Build history of the part. All positions in model axes, mm. A direction names the side the tool comes from. Coordinates: 2 decimals unless noted, no trailing zeros. Order: outer loops, then holes, each group sorted by start corner. A loop starts at its lowest first (then second) coordinate and runs counter-clockwise, first axis right, second up. Notation, with made-up numbers: (27.25, 27.25) - (43.25, 27.25) arc R8 ccw to (43.25, 38.25) - close; hole circle Ø1 at (67, 69.5). An arc over 180 degrees is marked (long way). Return JSON: item names as keys, results as strings.
from build123d import *

# Parameters (mm, degrees)
SKETCH1_R           = 2.3
BOSS_EXTRUDE1_DEPTH = 4
FILLET1_R           = 0.5
CHAMFER1_SIZE       = 0.5


with BuildPart() as part:
    # Sketch1 → Boss-Extrude1 (new body)
    with BuildSketch(Plane(origin=(0, 0, 0), x_dir=(1, 0, 0), z_dir=(0, 1, 0))):
        with Locations(Location((0, 0, 0), (0, 0, 270))):
            Circle(SKETCH1_R)
    extrude(amount=BOSS_EXTRUDE1_DEPTH)

    # Sketch2 → Revolve1 (revolve)
    with BuildSketch(Plane.XY, mode=Mode.PRIVATE) as revolve1_sk:
        with BuildLine():
            Line((-3, 5), (-3, 4))
            Line((-3, 4), (0, 4))
            Line((0, 4), (0, 7.16227766))
            ThreePointArc((0, 7.16227766), (-1.849016271, 6.565373039), (-3, 5))
        make_face()
    revolve(revolve1_sk.sketch.rotate(Axis((0, -2.040480146, 0), (0, 1, 0)), 180), axis=Axis((0, -2.040480146, 0), (0, 1, 0)))

    # Fillet1
    fillet1_edges = [part.edges().sort_by_distance(p)[0] for p in [
        (-3, 4, 0),
    ]]
    fillet(fillet1_edges, radius=FILLET1_R)

    # Chamfer1
    chamfer1_edges = [part.edges().sort_by_distance(p)[0] for p in [
        (0, 0, -2.3),
    ]]
    chamfer(chamfer1_edges, length=CHAMFER1_SIZE)


solid = part.part
1. Cut at B-B on x = 0. Give the cut face in (y, z).
Check values:
{"outline": "(0, -1.8) - (0.5, -2.3) - (4, -2.3) - (4, -2.5) arc R0.5 ccw to (4.5, -3) - (5, -3) arc R3.16 ccw to (5, 3) - (4.5, 3) arc R0.5 ccw to (4, 2.5) - (4, 2.3) - (0.5, 2.3) - (0, 1.8) - close"}
2. Drop flat-ended pins along their axis: pin 1 (3 mm diameter, centred on y = 1.5, z = 1.5, fed in from +X); pin 2 (1 mm diameter, centred on x = 2, z = 2, fed in from +Y); pin 3 (2 mm diameter, centred on x = -2.5, z = -2, fed in from +Y). Give the stop position or say it passes through.
Check values:
{"pin 1": "x = 2.3", "pin 2": "y = 6.14", "pin 3": "y = 6.27"}
3. Tool access for faces 1 (the flat face through (0, 0, 0)), 2 (the cylindrical face through (0.691, 2.226, 2.194)): list every direction of +Z, -Z, +X, -X, +Y, -Y with a clear straight run to the whole face (end or side of a thin tool).
Check values:
{"face 1": "+Z, -Z, +X, -X, -Y", "face 2": "-Y"}
4. Probe L1, parallel to X at y = 1.5, z = 0; L2, parallel to Y at x = -1.7, z = 1.15; L3, parallel to Z at x = 1.6, y = 2.75. List the from-to ranges inside material, lowest first.
Check values:
{"L1": "-2.3 to 2.3", "L2": "0.25 to 6.41", "L3": "-1.65 to 1.65"}
5. Cut at A-A on z = 0. Give the cut face in (x, y).
Check values:
{"outline": "(-3, 4.5) arc R0.5 ccw to (-2.5, 4) - (-2.3, 4) - (-2.3, 0.5) - (-1.8, 0) - (1.8, 0) - (2.3, 0.5) - (2.3, 4) - (2.5, 4) arc R0.5 ccw to (3, 4.5) - (3, 5) arc R3.16 ccw to (-3, 5) - close"}
6. Cut at C-C on y = 1. Give the cut face in (x, z).
Check values:
{"outline": "circle Ø4.6 at (0, 0)"}
